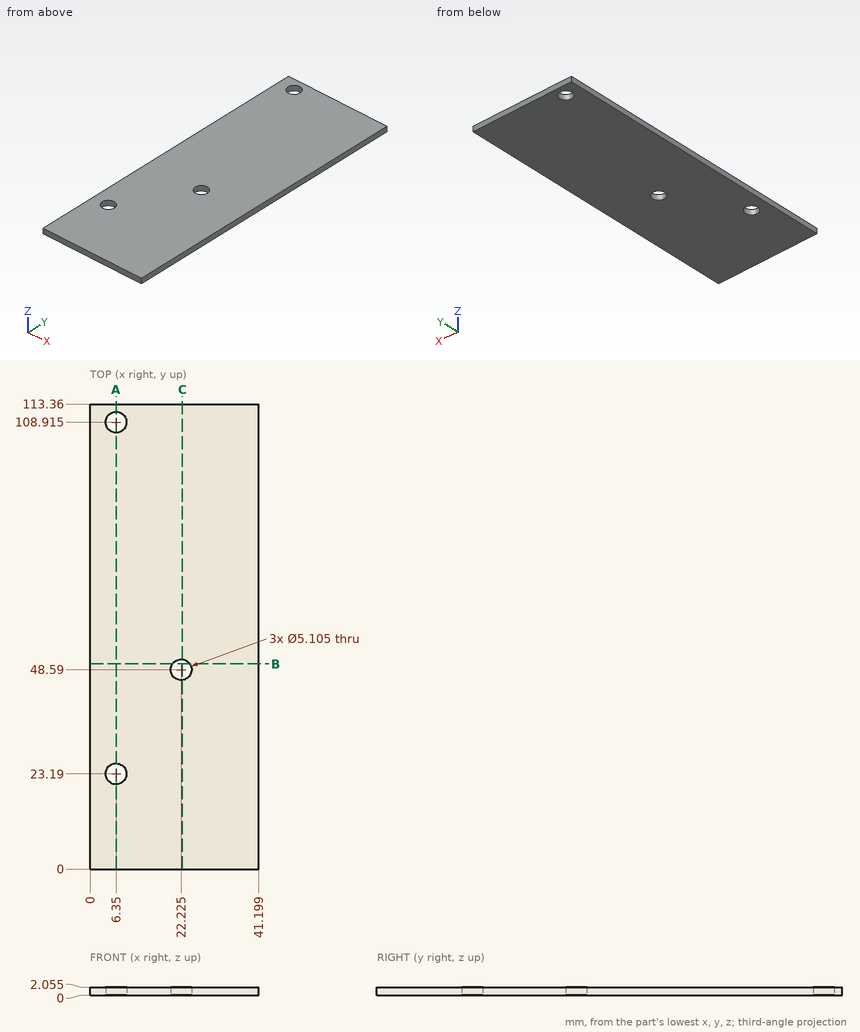
Geometry: see drawing. Coordinates: mm, zero at the bounding-box minimum. Coordinates: 2 decimals unless noted, no trailing zeros. Loops run counter-clockwise (first coordinate to the right, second up) from the corner with the lowest first, then second, coordinate; pieces in that order, holes last. Notation, with made-up numbers: (36.5, -17) - (44.5, -17) arc R35 ccw to (44.5, 22) - close; hole circle Ø5 at (7, 61.5). An arc over 180 degrees is marked (long way). Put each result on its own line as item: value. Start each with the question number.
Q1. Cut plane B-B, the plane y = 50. Return loops of the section in (x, z) (1 decimal).
Q2. Line query: line 1 (Y direction, x = 6.35, z = 1.1); line 2 (Y direction, x = 4, z = 0.6) (1 decimal); line 3 (Y direction, x = 20, z = 0.8) (1 decimal). Output: solid intervals per line, ascending.
Q3. Cut plane A-A, the plane x = 6.35. Return loops of the section in (y, z) (1 decimal), and give its area (3 significant figures).
Q4. Pin query (flat end, axial travel): pin 1 Ø4 at (x, y) = (6.35, 23.19) entering from -Z (3 decimals). Return the tip coordinate at first contact, or that it passes through.
Q5. Cut plane C-C, the plane x = 22.5. Return loops of the section in (y, z) (1 decimal).
Filled sheet:
1. outline: (0, 0) - (20.1, 0) - (20.1, 2.1) - (0, 2.1) - close; (24.4, 0) - (41.2, 0) - (41.2, 2.1) - (24.4, 2.1) - close
2. line 1: 0 to 20.64, 25.74 to 106.36, 111.47 to 113.36
2. line 2: 0 to 22.2, 24.2 to 107.9, 109.9 to 113.4
2. line 3: 0 to 47.3, 49.8 to 113.4
3. outline: (0, 0) - (20.6, 0) - (20.6, 2.1) - (0, 2.1) - close; (25.7, 0) - (106.4, 0) - (106.4, 2.1) - (25.7, 2.1) - close; (111.5, 0) - (113.4, 0) - (113.4, 2.1) - (111.5, 2.1) - close
3. area: 212 mm²
4. pin 1: through
5. outline: (0, 0) - (46.1, 0) - (46.1, 2.1) - (0, 2.1) - close; (51.1, 0) - (113.4, 0) - (113.4, 2.1) - (51.1, 2.1) - close
